Can you work these out from the drawing? Everything is in mm from the part's minimum corner. Round coordinates to 2 decimals unless told otherwise and drop trailing zeros. Write each loop counter-clockwise with the first axis right and the second up, starting at its lowest first coordinate (ties: lowest second). Pieces come first, ordered by that corner, then holes.
Q1. If we section it at A-A (z = 57.5): Please give me the cut outline in (x, y).
Q2. If we section it at C-C (y = 94): Please give me the cut outline in (x, z), plus the area to 3 significant figures.
Q3. Please list where these lines run through material, in increasing order: line 1 along Y through (x, z) = (63, 81.5); line 2 along X through (y, z) = (47, 43); line 3 along Y through (x, z) = (7, 11.5).
Q4. If we section it at D-D (z = 116.5): Please give me the cut outline in (x, y).
Q5. If we section it at B-B (x = 50): Please give me the cut outline in (y, z), plus the area to 3 significant figures.
Q6. I'm going to push flat-ended pins straight in: pin 1 Ø3 at (y, z) = (70.5, 110.5) entering from +X; pin 2 Ø2 at (x, z) = (101.5, 83) entering from -Y; pin 3 Ø3 at (x, z) = (54, 32) entering from +Y. Where does each tip first touch, or does it pass through?
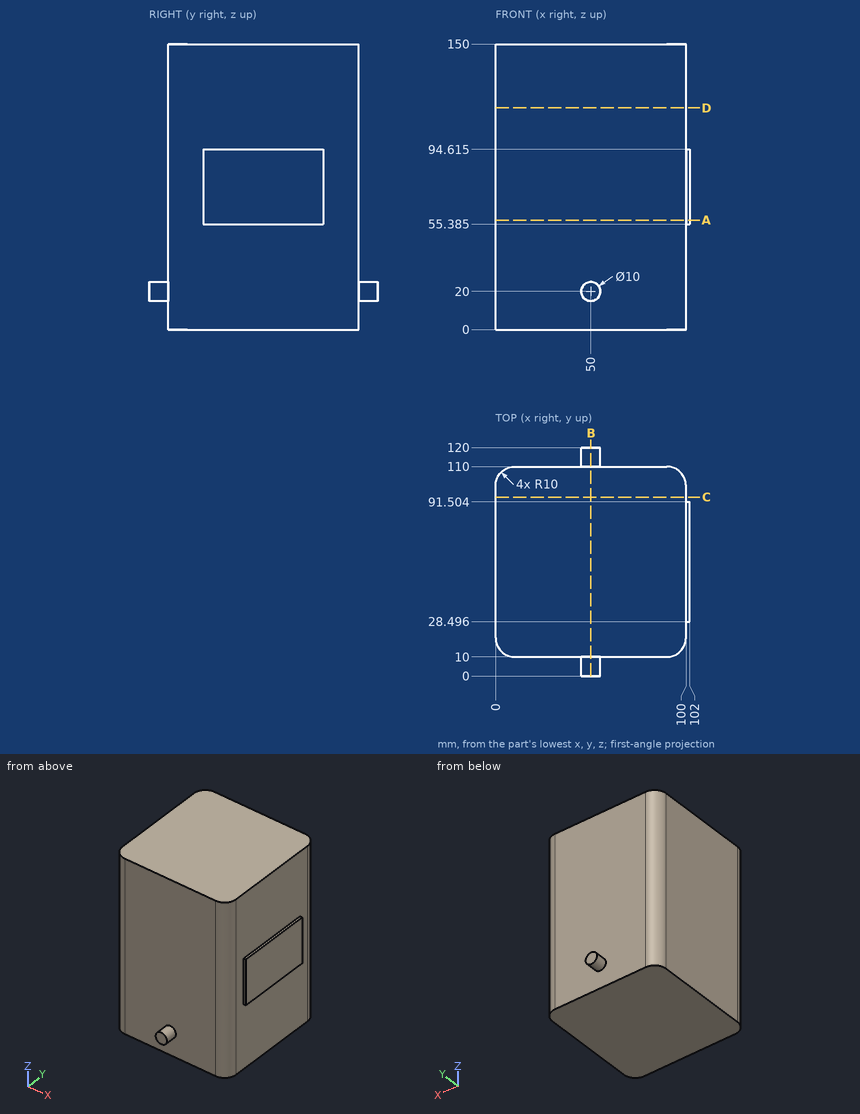
A:
1. outline: (0, 20) arc R10 ccw to (10, 10) - (90, 10) arc R10 ccw to (100, 20) - (100, 28.5) - (102, 28.5) - (102, 91.5) - (100, 91.5) - (100, 100) arc R10 ccw to (90, 110) - (10, 110) arc R10 ccw to (0, 100) - close
2. outline: (0, 0) - (100, 0) - (100, 150) - (0, 150) - close
2. area: 15,000 mm2
3. line 1: y = 10 to 110
3. line 2: x = 0 to 100
3. line 3: y = 10.46 to 109.54
4. outline: (0, 20) arc R10 ccw to (10, 10) - (90, 10) arc R10 ccw to (100, 20) - (100, 100) arc R10 ccw to (90, 110) - (10, 110) arc R10 ccw to (0, 100) - close
5. outline: (0, 15) - (10, 15) - (10, 0) - (110, 0) - (110, 15) - (120, 15) - (120, 25) - (110, 25) - (110, 150) - (10, 150) - (10, 25) - (0, 25) - close
5. area: 15,200 mm2
6. pin 1: stops at x = 100
6. pin 2: stops at y = 28.5
6. pin 3: stops at y = 110
